Job drawing, mm, ordinate dimensions from the low corner. One solid piece. A direction names the side the tool comes from. Coordinates: 2 decimals unless noted, no trailing zeros. Order: outer loops, then holes, each group sorted by start corner. A loop starts at its lowest first (then second) coordinate and runs counter-clockwise, first axis right, second up. Notation, with made-up numbers: (26.5, 89) - (43.5, 89) arc R25 ccw to (43.5, 126) - close; hole circle Ø5 at (39.25, 82). An arc over 180 degrees is marked (long way). Return JSON: item names as keys, results as strings.
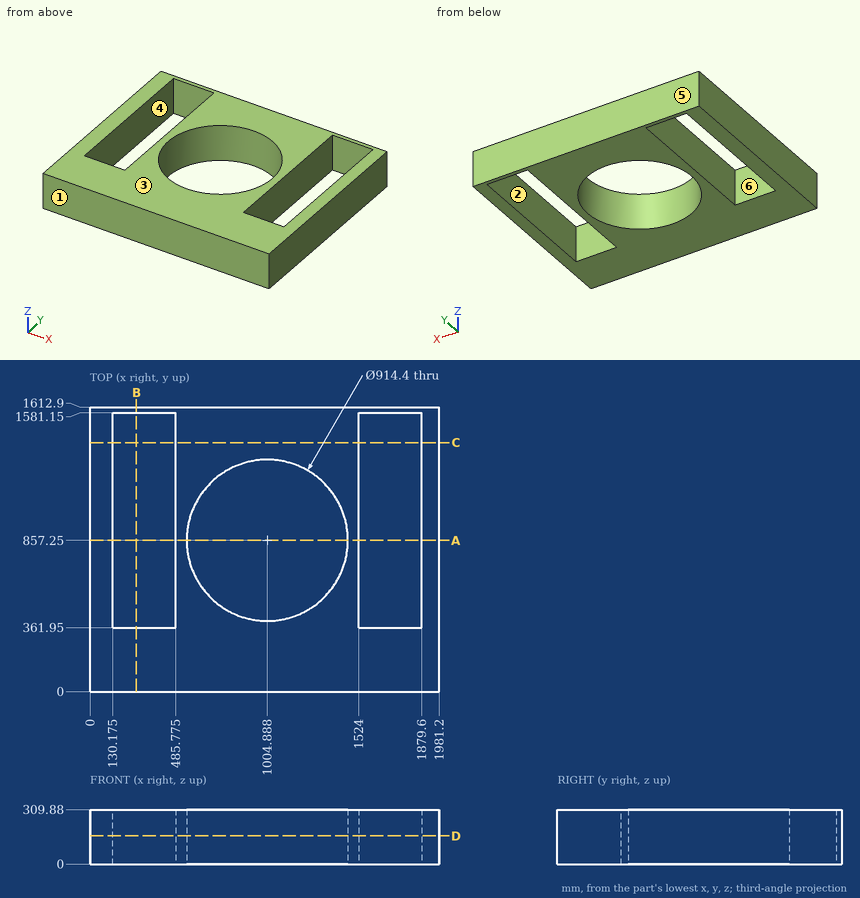
1. Probe L1, parallel to X at y = 857, z = 187 (1 decimal); L2, parallel to Y at x = 234.5, z = 202; L3, parallel to X at y = 626.5, z = 277 (1 decimal). List the from-to ranges inside material, lowest first.
Check values:
{"L1": "0 to 130.2, 485.8 to 547.7, 1462.1 to 1524, 1879.6 to 1981.2", "L2": "0 to 361.95, 1581.15 to 1612.9", "L3": "0 to 130.2, 485.8 to 610.2, 1399.6 to 1524, 1879.6 to 1981.2"}
2. Cut at D-D on z = 160. State how many separate pieces and enclosed holes the cut face has, plus the area to 3 significant figures.
Check values:
{"separate pieces": "1", "enclosed holes": "3", "area": "1,670,000 mm²"}
3. Cut at A-A on y = 857.25. Give the cut face in (x, z) (1 decimal), plus the area to 3 significant figures.
Check values:
{"outline": "(0, 0) - (130.2, 0) - (130.2, 309.9) - (0, 309.9) - close; (485.8, 0) - (547.7, 0) - (547.7, 309.9) - (485.8, 309.9) - close; (1462.1, 0) - (1524, 0) - (1524, 309.9) - (1462.1, 309.9) - close; (1879.6, 0) - (1981.2, 0) - (1981.2, 309.9) - (1879.6, 309.9) - close", "area": "110,000 mm²"}
4. Mould opens along Y. For the marked faces 1, 2, 3 and 4 say: pulls with the +Y half, pulls with the -Y half, needs draft (parallel to the pull), parting line crosses it, or undercut.
Check values:
{"face 1": "pulls with the -Y half", "face 2": "undercut", "face 3": "needs draft", "face 4": "undercut"}
5. Cut at B-B on x = 262.5. Give the cut face in (y, z).
Check values:
{"outline": "(0, 0) - (361.95, 0) - (361.95, 309.88) - (0, 309.88) - close; (1581.15, 0) - (1612.9, 0) - (1612.9, 309.88) - (1581.15, 309.88) - close"}
6. Tool access for the marked faces 5 and 6: list every direction of +Z, -Z, +X, -X, +Y, -Y with a clear straight run to the whole face (end or side of a thin tool).
Check values:
{"face 5": "+Z, -Z, +X, -X, +Y", "face 6": "+Z, -Z"}
7. Cut at C-C on y = 1410.5. Give the cut face in (x, z) (1 decimal).
Check values:
{"outline": "(0, 0) - (130.2, 0) - (130.2, 309.9) - (0, 309.9) - close; (485.8, 0) - (1524, 0) - (1524, 309.9) - (485.8, 309.9) - close; (1879.6, 0) - (1981.2, 0) - (1981.2, 309.9) - (1879.6, 309.9) - close"}
